Verification items for the finished model (mm, model axes). Give positions to 0.01 mm unless a question says otherwise; leave off trailing zeros. Loops run counter-clockwise (first coordinate to the right, second up) from the corner with the lowest first, then second, coordinate; pieces in that order, holes last. Notation, with made-up numbers: (28, 48.25) - (32, 48.25) arc R6 ccw to (32, 58.25) - close; hole circle Ø7 at (-9, 48.5). An arc over 180 degrees is marked (long way). One line per question, with ' | ' between items. Start each with the question number.
1. Depth check by flat-ended pin: pin 1 Ø2 at (x, z) = (-40, 5) entering from -Y; pin 2 Ø3 at (y, z) = (90, 2.5) entering from +X; pin 3 Ø1.7 at (x, y) = (130.175, -38.1) entering from +Z. Enter the tip coordinate at first touch or a pass-through.
2. Thickness scan on line 1 along Y through (x, z) = (-114.3, 1.5); line 2 along X through (y, z) = (45, 3.5); line 3 along Y through (x, z) = (-122.5, 3). Record the ranges inside material, lowest first. Write a range as from..to.
3. Section check B-B, the plane y = -55.88. Enter the section's corners in (x, z).
4. Mould release check, pull along Y, two halves, no side actions. Record for faces 1 (the face through (9.052, -51.945, 3.131)), 2 (the face through (-3, 24, 6.35)): +Y half, -Y half, draft (parallel to the pull), parting line (faces both ways), or undercut.
5. Section check A-A, the plane x = -32. Enter the section's corners in (y, z), then the cut area to 3 significant figures.
6. Section check C-C, the plane x = 69. Enter the section's corners in (y, z).
7. Section check D-D, the plane z = 3.25. State how many separate pieces and enclosed holes the cut face has, then the cut area to 3 significant figures.
from build123d import *

# Parameters (mm, degrees)
SKETCH1_W                            = 393.7
SKETCH1_H                            = 127
BOSS_EXTRUDE1_DEPTH                  = 6.35
BOSS_EXTRUDE2_DEPTH                  = 6.35
FILLET1_R                            = 6.35
SKETCH11_W                           = 95.25
SKETCH11_H                           = 25.4
CUT_EXTRUDE1_DEPTH                   = 226.28847424
F_5_16_0_3125_DIAMETER_HOLE1_D       = 7.9375
F_11_64_0_17188_DIAMETER_HOLE1_D     = 4.365752
F_35_0_11_DIAMETER_HOLE1_D           = 2.794
F_35_0_11_DIAMETER_HOLE1_DEPTH       = 8.89
F_35_0_11_DIAMETER_HOLE1_TIP         = 0.839402285
F_11_64_0_17188_DIAMETER_HOLE2_D     = 4.365752
F_11_64_0_17188_DIAMETER_HOLE2_DEPTH = 8.89
F_11_64_0_17188_DIAMETER_HOLE2_TIP   = 1.311604225


with BuildPart() as part:
    # Sketch1 → Boss-Extrude1 (new body)
    with BuildSketch(Plane.XY):
        Rectangle(SKETCH1_W, SKETCH1_H)
    extrude(amount=BOSS_EXTRUDE1_DEPTH)

    # Sketch10 → Boss-Extrude2 (add)
    with BuildSketch(Plane.XY.offset(6.35)):
        Polygon((-152.4, 96.68304999), (-152.4, 63.5), (-139.7, 63.5), (-139.7, 96.68304999), (0, 96.68304999), (0, 109.38304999), (-146.05, 109.38304999), (-152.4, 109.38304999), align=None)
        Polygon((139.7, 96.68304999), (139.7, 63.5), (152.4, 63.5), (152.4, 109.38304999), (0, 109.38304999), (0, 96.68304999), align=None)
    extrude(amount=-BOSS_EXTRUDE2_DEPTH)

    # Fillet1
    fillet1_edges = [part.edges().sort_by_distance(p)[0] for p in [
        (139.7, 96.68304999, 3.175),
        (-139.7, 96.68304999, 3.175),
        (-139.7, 63.5, 3.175),
        (-152.4, 63.5, 3.175),
        (-152.4, 109.38304999, 3.175),
        (152.4, 109.38304999, 3.175),
        (152.4, 63.5, 3.175),
        (139.7, 63.5, 3.175),
    ]]
    fillet(fillet1_edges, radius=FILLET1_R)

    # Sketch11 → Cut-Extrude1 (cut, through all)
    with BuildSketch(Plane.XY.offset(6.35)):
        with Locations((-53.975, -50.8)):
            Rectangle(SKETCH11_W, SKETCH11_H)
    extrude(amount=-CUT_EXTRUDE1_DEPTH, mode=Mode.SUBTRACT)

    # 5/16 (0.3125) Diameter Hole1 (through all)
    with Locations(Plane.XY.offset(6.35)):
        with Locations((8.534908, -55.88)):
            Hole(F_5_16_0_3125_DIAMETER_HOLE1_D / 2)

    # 11/64 (0.17188) Diameter Hole1 (through all)
    with Locations(Plane.XY.offset(6.35)):
        with Locations((-114.3, 44.45), (-114.3, 19.05), (-114.3, -6.35), (114.3, 44.45), (114.3, 19.05), (114.3, -6.35)):
            Hole(F_11_64_0_17188_DIAMETER_HOLE1_D / 2)

    # #35 (0.11) Diameter Hole1
    with Locations(Plane.XY.offset(6.35)):
        with Locations((-193.675, 38.1), (-130.175, 38.1), (-130.175, 0), (-193.675, 0), (-193.675, -38.1), (-130.175, -38.1), (130.175, -38.1), (193.675, -38.1), (193.675, 0), (193.675, 38.1), (130.175, 38.1), (130.175, 0)):
            Hole(F_35_0_11_DIAMETER_HOLE1_D / 2, depth=F_35_0_11_DIAMETER_HOLE1_DEPTH)
            with Locations((0, 0, -(F_35_0_11_DIAMETER_HOLE1_DEPTH + F_35_0_11_DIAMETER_HOLE1_TIP / 2))):  # 118° drill point
                Cone(0, F_35_0_11_DIAMETER_HOLE1_D / 2, F_35_0_11_DIAMETER_HOLE1_TIP, mode=Mode.SUBTRACT)

    # 11/64 (0.17188) Diameter Hole2
    with Locations(Plane.XY.offset(6.35)):
        with Locations((0, 19.05)):
            Hole(F_11_64_0_17188_DIAMETER_HOLE2_D / 2, depth=F_11_64_0_17188_DIAMETER_HOLE2_DEPTH)
            with Locations((0, 0, -(F_11_64_0_17188_DIAMETER_HOLE2_DEPTH + F_11_64_0_17188_DIAMETER_HOLE2_TIP / 2))):  # 118° drill point
                Cone(0, F_11_64_0_17188_DIAMETER_HOLE2_D / 2, F_11_64_0_17188_DIAMETER_HOLE2_TIP, mode=Mode.SUBTRACT)


solid = part.part
Results list:
1) pin 1: y = -38.1 | pin 2: x = 152.4 | pin 3: through
2) line 1: -63.5..-8.53, -4.17..16.87, 21.23..42.27, 46.63..63.5, 96.68..109.38 | line 2: -196.85..-116.41, -112.19..112.19, 116.41..196.85 | line 3: -63.5..63.5, 96.68..109.38
3) outline: (-196.85, 0) - (-101.6, 0) - (-101.6, 6.35) - (-196.85, 6.35) - close; (-6.35, 0) - (4.57, 0) - (4.57, 6.35) - (-6.35, 6.35) - close; (12.5, 0) - (196.85, 0) - (196.85, 6.35) - (12.5, 6.35) - close
4) face 1: undercut | face 2: draft
5) outline: (-38.1, 0) - (63.5, 0) - (63.5, 6.35) - (-38.1, 6.35) - close; (96.68, 0) - (109.38, 0) - (109.38, 6.35) - (96.68, 6.35) - close | area: 726 mm²
6) outline: (-63.5, 0) - (63.5, 0) - (63.5, 6.35) - (-63.5, 6.35) - close; (96.68, 0) - (109.38, 0) - (109.38, 6.35) - (96.68, 6.35) - close
7) separate pieces: 1 | enclosed holes: 21 | area: 52,100 mm²
